```python
from build123d import *

# Parameters (mm, degrees)
SKETCH1_W              = 42.672
SKETCH1_H              = 38.1
BOSS_EXTRUDE1_DEPTH    = 38.1
SKETCH3_R              = 3.175
CUT_EXTRUDE1_DEPTH     = 69.732231042
FILLET1_R              = 6
SPLIT1_START           = -38.1
SPLIT1_OUTLINE_R       = 3.175
SPLIT1_DEPTH           = 38.1
SPLIT2_SURFACE_1_BACK  = 69.732
SPLIT2_SURFACE_1_DEPTH = 139.464


# Read off the part's stored shape, not the designer's step: Split1
with BuildPart() as part:
    # Sketch1 → Boss-Extrude1 (new body)
    with BuildSketch(Plane(origin=(0, 0, 0), x_dir=(1, 0, 0), z_dir=(0, 1, 0))):
        with Locations((21.336, 19.05)):
            Rectangle(SKETCH1_W, SKETCH1_H)
    extrude(amount=BOSS_EXTRUDE1_DEPTH)

    # Sketch3 → Cut-Extrude1 (cut, through all)
    with BuildSketch(Plane(origin=(0, 0, 0), x_dir=(1, 0, 0), z_dir=(0, 1, 0))):
        with Locations(Location((10.922, 19.05, 0), (0, 0, 90))):
            Circle(SKETCH3_R)
        with Locations(Location((33.02, 19.05, 0), (0, 0, 90))):
            Circle(SKETCH3_R)
    extrude(amount=CUT_EXTRUDE1_DEPTH, mode=Mode.SUBTRACT)

    # Fillet1
    fillet1_edges = [part.edges().sort_by_distance(p)[0] for p in [
        (42.672, 19.05, -38.1),
        (42.672, 19.05, 0),
    ]]
    fillet(fillet1_edges, radius=FILLET1_R)

    # Split1 outline → Split1 (cut)
    with BuildSketch(Plane.XY.offset(SPLIT1_START)):
        with Locations((10.922, 27.178)):
            Circle(SPLIT1_OUTLINE_R)
        with BuildLine():
            ThreePointArc((21.844, 27.178), (27.140915284, 14.390115284), (39.9288, 9.0932))
            Line((39.9288, 9.0932), (42.672, 9.0932))
            Line((42.672, 9.0932), (42.672, 38.1))
            Line((42.672, 38.1), (10.922, 38.1))
            ThreePointArc((10.922, 38.1), (18.645020264, 34.901020264), (21.844, 27.178))
        make_face()
        with BuildLine():
            ThreePointArc((0, 27.178), (3.198979736, 34.901020264), (10.922, 38.1))
            Line((10.922, 38.1), (0, 38.1))
            Line((0, 38.1), (0, 27.178))
        make_face()
    extrude(amount=SPLIT1_DEPTH, mode=Mode.SUBTRACT)

    # Split2: cut with a surface, the side behind it stays
    # Split2 surface: a surface, the sketch's curves swept straight by 139.464 mm
    with BuildLine(Plane(origin=(42.672, 0, 0), x_dir=(0, 0, -1), z_dir=(1, 0, 0)).offset(-SPLIT2_SURFACE_1_BACK), mode=Mode.PRIVATE) as split2_surface_1_path:
        Line((9.0932, 38.1), (9.0932, 9.0932))
        Line((9.0932, 9.0932), (29.0068, 9.0932))
        Line((29.0068, 9.0932), (29.0068, 38.1))
    split2_surface_1 = Shell.extrude(split2_surface_1_path.wire(), (1 * SPLIT2_SURFACE_1_DEPTH, 0 * SPLIT2_SURFACE_1_DEPTH, 0 * SPLIT2_SURFACE_1_DEPTH))
    split(bisect_by=split2_surface_1, keep=Keep.BOTTOM)


solid = part.part
```
Could you check a few things on this model? Use its own coordinates, in mm. A direction names the side the tool comes from. Round coordinates to 2 decimals unless told otherwise and drop trailing zeros. Order: outer loops, then holes, each group sorted by start corner. A loop starts at its lowest first (then second) coordinate and runs counter-clockwise, first axis right, second up. Notation, with made-up numbers: (-11, 18) -> (18, 18) arc R11 ccw to (18, 33) -> close; hole circle Ø10 at (7.5, 71). An arc over 180 degrees is marked (long way). One line per question, with ' | ' between items.
Q1. If we section it at C-C on z = -8: Write out the boundary of the cut face in (x, y) (3 decimals).
Computed values:
outline: (0, 0) -> (42.672, 0) -> (42.672, 9.093) -> (39.929, 9.093) arc R18.085 cw to (21.844, 27.178) arc R10.922 ccw to (0, 27.178) -> close; hole circle Ø6.35 at (10.922, 27.178)
Q2. If we section it at D-D on y = 26: Write out the boundary of the cut face in (x, z).
Computed values:
outline: (0, -38.1) -> (7.97, -38.1) -> (7.97, -29.01) -> (0, -29.01) -> close; (0, -9.09) -> (7.97, -9.09) -> (7.97, 0) -> (0, 0) -> close; (13.87, -38.1) -> (21.88, -38.1) -> (21.88, -29.01) -> (13.87, -29.01) -> close; (13.87, -9.09) -> (21.88, -9.09) -> (21.88, 0) -> (13.87, 0) -> close
Q3. If we section it at B-B on y = 11: Write out the boundary of the cut face in (x, z).
Computed values:
outline: (0, -38.1) -> (31.85, -38.1) -> (31.85, -29.01) -> (0, -29.01) -> close; (0, -9.09) -> (31.85, -9.09) -> (31.85, 0) -> (0, 0) -> close
Q4. I'm going to push flat-ended pins straight in: pin 1 (1.5 mm diameter, centred on x = 23, z = -27, fed in from +Y); pin 2 (5 mm diameter, centred on x = 10.922, y = 27.178, fed in from -Z); pin 3 (12 mm diameter, centred on x = 26, z = -19.5, fed in from -Y); pin 4 (2 mm diameter, centred on x = 38, y = 10, fed in from +Z). Where does each tip first touch, or does it pass through?
Computed values:
pin 1: y = 9.09 | pin 2: through | pin 3: y = 0 | pin 4: z = -0.03
Q5. If I drill on line 1 (Z direction, x = 6, y = 16); line 2 (X direction, y = 3, z = -19.05) (3 decimals); line 3 (Z direction, x = 33, y = 3), over which ranges is the centre line in solid material (lowest first)? Write a range as from..to.
Computed values:
line 1: -38.1..-29.01, -9.09..0 | line 2: 0..7.747, 14.097..29.845, 36.195..42.672 | line 3: -38.1..-22.22, -15.88..0
Q6. We'd pull the mould along X, two halves only. Please class faces 1 (the face through (14, 15, -38.1)), 2 (the face through (8.4, 25.25, -33.62)), 3 (the face through (0, 7, -19)): released by +X, released by -X, zero draft, split by the parting line, or undercut.
Computed values:
face 1: zero draft | face 2: undercut | face 3: released by -X
Q7. If we section it at A-A on z = -19.05: Write out the boundary of the cut face in (x, y) (3 decimals).
Computed values:
outline: (0, 0) -> (7.747, 0) -> (7.747, 9.093) -> (0, 9.093) -> close; (14.097, 0) -> (29.845, 0) -> (29.845, 9.093) -> (14.097, 9.093) -> close; (36.195, 0) -> (42.672, 0) -> (42.672, 9.093) -> (36.195, 9.093) -> close
Q8. Which directions (+Z, -Z, +X, -X, +Y, -Y) give clear straight access to the entire face, cutting with the end or side of a thin tool? Please do faces 4 (the face through (10.78, 4.48, -15.88)), 5 (the face through (11, 21, -9.093)).
Computed values:
face 4: +Y, -Y | face 5: +X, -X, +Y
